Autodesk Inventor part; units mm, degrees
ref_plane "YZ Plane" through (0, 0, 0) normal (1, 0, 0) x (0, 1, 0)
ref_plane "XZ Plane" through (0, 0, 0) normal (0, 1, 0) x (-1, 0, 0)
ref_plane "XY Plane" through (0, 0, 0) normal (0, 0, 1) x (1, 0, 0)
sketch "Sketch1" plane through (0, 0, 0) normal (0, 1, 0) x (-1, 0, 0)
  circle A0 centre (0, 0) radius 3.55
  circle A1 centre (0, 0) radius 2.8
  line L0 (0, -2.8) -> (0, -1.9)
  line L1 (0, 2.8) -> (0, 1.9)
  line L2 (2.0567, 1.9) -> (-2.0567, 1.9)
  line L3 (-2.0567, -1.9) -> (2.0567, -1.9)
  dimension "d0" = 7.1
  dimension "d1" = 5.6
  dimension "d2" = 0.9
  dimension "d3" = 0.9
  dimension "d4" = 4.1134
  dimension "d5" = 4.1134
extrude "Extrusion1" add sketch "Sketch1" along normal blind 8.5 contours A0 | L2 L1 A1 | A1 L0 L3 | L1 L2 A1 | A1 L3 L0
sketch "Sketch2" plane through (0, 8.5, 0) normal (0, 1, 0) x (1, 0, 0)
  arc A0 (-2.0567, 1.9) -> (-2.0567, -1.9) centre (0, 0) ccw
  circle A1 centre (0, 0) radius 3.55
  dimension "d8" = 7.1
extrude "Extrusion2" add sketch "Sketch2" along normal blind 11.5
sketch "Sketch3" plane through (0, 0, 0) normal (0, 0, 1) x (1, 0, 0)
  line L0 (3.55, 20) -> (-3.55, 20) construction
  line L1 (0, 20) -> (0, 32) construction
  line L2 (0, 32) -> (-12, 32) construction
  line L3 (0, 32) -> (12, 32) construction
  arc A0 (-12, 32) -> (-3.55, 20) centre (0.4988, 31.8261) ccw
  arc A1 (3.55, 20) -> (12, 32) centre (-0.4988, 31.8261) ccw
  line L4 (-12, 32) -> (-8, 32)
  line L5 (12, 32) -> (8, 32)
  circle A2 centre (0, 32) radius 8
  line L6 (-12, 32) -> (-8, 32)
  line L7 (-8, 32) -> (-8, 39)
  line L8 (-8, 39) -> (-12, 39)
  line L9 (-12, 39) -> (-12, 32)
  line L10 (12, 32) -> (8, 32)
  line L11 (8, 32) -> (8, 39)
  line L12 (8, 39) -> (12, 39)
  line L13 (12, 39) -> (12, 32)
  line L14 (-8, 32) -> (-8, 34.0142) construction
  line L15 (-8, 39) -> (-8, 37.5) construction
  line L16 (8, 32) -> (8, 35.1588) construction
  line L17 (-8, 37.5) -> (8, 37.5)
  line L18 (8, 37.5) -> (8, 33.5)
  line L19 (8, 33.5) -> (-8, 33.5)
  line L20 (-8, 33.5) -> (-8, 37.5)
  line L21 (-3.55, 20) -> (3.55, 20)
  point P0 (0, 0)
  point P1 (8, 37.5)
  dimension "d11" = 12
  dimension "d12" = 12
  dimension "d13" = 12
  dimension "d14" = 12.5
  dimension "d15" = 12.5
  dimension "d16" = 4
  dimension "d17" = 4
  dimension "d18" = 7
  dimension "d19" = 7
  dimension "d20" = 4
  dimension "d21" = 4
  dimension "d22" = 1.5
  dimension "d23" = 1.5
  dimension "d24" = 1.5
extrude "Extrusion3" add sketch "Sketch3" along normal mid plane 10 contours L4 A2 L5 A1 L21 A0 | L9 L8 L7 L4 | L11 L12 L13 L5 | L19 L7 L17 A2 | A2 L17 L19 | A2 L17 L11 L19
sketch "Sketch4" plane through (-8, 37.5, 5) normal (0, 1, 0) x (1, 0, 0)
  circle A0 centre (8, 5) radius 3.55
  circle A1 centre (8, 5) radius 3.55
  point P0 (8, 3.5)
extrude "Extrusion4" cut sketch "Sketch4" against normal blind 10
properties part number "Universal joint"
Part model, mm, in its own coordinate system. A direction names the side the tool comes from. Give positions to 0.01 mm unless a question says otherwise; leave off trailing zeros. Order: outer loops, then holes, each group sorted by start corner. A loop starts at its lowest first (then second) coordinate and runs counter-clockwise, first axis right, second up. Notation, with made-up numbers: (63.25, 70.25) - (110.25, 70.25) arc R18 ccw to (110.25, 94.25) - close; hole circle Ø11 at (6, 3). An arc over 180 degrees is marked (long way). Use a Markdown table: item, result.
1) Two-plate mould, pull along Z, no slides. Class faces 6 (the flat face through (0, 34, 5)), 7 (the flat face through (-10, 39, 0)), 8 (the cylindrical face through (-0.46, 35.53, -3.52)): +Z half, -Z half, draft (parallel to the pull), parting line (faces both ways), or undercut.
Checked values:
| item | result |
|---|---|
| face 6 | +Z half |
| face 7 | draft |
| face 8 | undercut |
2) Flat gauge pins, fed straight in: P1, Ø3, axis at x = -1.5, z = 2, coming from the +Y side; P2, Ø1, axis at y = 15, z = 0.5, coming from the +X side; P3, Ø2, axis at x = 0, y = 6, coming from the -Z side. Where does each tip first touch, or does it go through?
Checked values:
| item | result |
|---|---|
| P1 | y = 37.5 |
| P2 | x = 3.55 |
| P3 | z = -3.55 |
3) Saw through at D-D on y = 5.5. List the corners of the cut face in (x, z), plus the area to 3 significant figures.
Checked values:
| item | result |
|---|---|
| outline | circle Ø7.1 at (0, 0); hole (-2.06, -1.9) - (2.06, -1.9) arc R2.8 ccw to (2.06, 1.9) - (-2.06, 1.9) arc R2.8 ccw to start |
| area | 20.1 mm² |
4) Saw through at B-B on y = 29. List the corners of the cut face in (x, z).
Checked values:
| item | result |
|---|---|
| outline | (-11.68, -5) - (-7.42, -5) - (-7.42, 5) - (-11.68, 5) - close; (7.42, -5) - (11.68, -5) - (11.68, 5) - (7.42, 5) - close |
5) Probe L1, parallel to X at y = 34.6, z = 0; L2, parallel to Z at x = 0, y = 34.4; L3, parallel to X at y = 33, z = 1.75. List the from-to ranges inside material, lowest first. Write a range as from..to.
Checked values:
| item | result |
|---|---|
| L1 | -12..-3.55, 3.55..12 |
| L2 | -5..-3.55, 3.55..5 |
| L3 | -12..-8, 8..12 |
6) 3-axis set-ups, long thin cutter, end or side, ignore diameter. For faces 1 (the flat face through (12, 36, 0)), 2 (the cylindrical face through (2.8, 4.2, 0)), 3 (the flat face through (8, 33, 0)), 4 (the flat face through (-4, 37.5, 0)), 5 (the flat face through (0, 34, -5)): which of +Z, -Z, +X, -X, +Y, -Y reach the whole face in a straight line?
Checked values:
| item | result |
|---|---|
| face 1 | +Z, -Z, +X, +Y, -Y |
| face 2 | -Y |
| face 3 | +Z, -Z |
| face 4 | +Z, -Z, +Y |
| face 5 | -Z, +X, -X, +Y, -Y |
7) Saw through at C-C on x = -7.5. List the corners of the cut face in (y, z), plus the area to 3 significant figures.
Checked values:
| item | result |
|---|---|
| outline | (22.22, -5) - (29.22, -5) - (29.22, 5) - (22.22, 5) - close; (33.5, -5) - (37.5, -5) - (37.5, 5) - (33.5, 5) - close |
| area | 110 mm² |
8) Saw through at A-A on x = 0. List the corners of the cut face in (y, z).
Checked values:
| item | result |
|---|---|
| outline | (0, -3.55) - (20, -3.55) - (20, -5) - (24, -5) - (24, 5) - (20, 5) - (20, 3.55) - (0, 3.55) - (0, 1.9) - (8.5, 1.9) - (8.5, -1.9) - (0, -1.9) - close; (33.5, -5) - (37.5, -5) - (37.5, -3.55) - (33.5, -3.55) - close; (33.5, 3.55) - (37.5, 3.55) - (37.5, 5) - (33.5, 5) - close |
